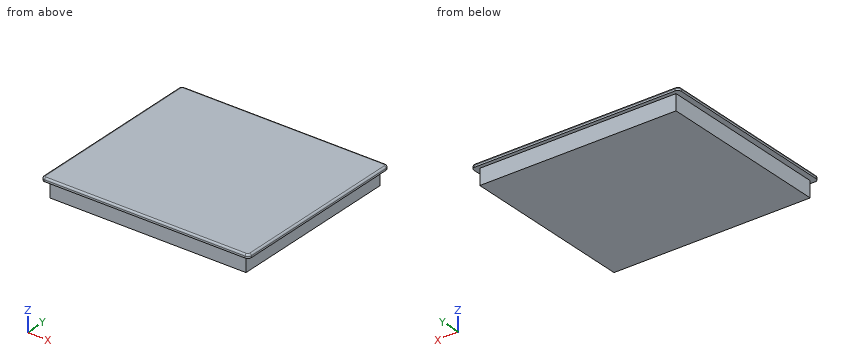
```python
from build123d import *

# Parameters (mm, degrees)
F0_W     = 560
F0_H     = 500
F1_DEPTH = 55
F2_DEPTH = 10
F3_R     = 5


with BuildPart() as f1:
    # F0 (on Top) → F1 (new body)
    with BuildSketch(Plane.XY):
        Rectangle(F0_W, F0_H)
    extrude(amount=-F1_DEPTH)

    # F0 (on Top) → F2 (join)
    with BuildSketch(Plane.XY):
        with BuildLine():
            Line((286, 261), (-286, 261))
            ThreePointArc((-286, 261), (-293.071068, 258.071068), (-296, 251))
            Line((-296, 251), (-296, -251))
            ThreePointArc((-296, -251), (-293.071068, -258.071068), (-286, -261))
            Line((-286, -261), (286, -261))
            ThreePointArc((286, -261), (293.071068, -258.071068), (296, -251))
            Line((296, -251), (296, 251))
            ThreePointArc((296, 251), (293.071068, 258.071068), (286, 261))
        make_face()
        Rectangle(F0_W, F0_H, mode=Mode.SUBTRACT)
        Rectangle(F0_W, F0_H)
    extrude(amount=-F2_DEPTH)

    # F3
    f3_edges = [f1.edges().sort_by_distance(p)[0] for p in [
        (0, 261, 0),
        (-293.071068, 258.071068, 0),
        (-296, 0, 0),
        (-293.071068, -258.071068, 0),
        (0, -261, 0),
        (293.071068, -258.071068, 0),
        (296, 0, 0),
        (293.071068, 258.071068, 0),
    ]]
    fillet(f3_edges, radius=F3_R)


solid = f1.part
```
For this review, take the finished solid that the model builds, in its own axes (mm). Round coordinates to 2 decimals unless told otherwise and drop trailing zeros. Write each loop counter-clockwise with the first axis right and the second up, starting at its lowest first coordinate (ties: lowest second). Pieces come first, ordered by that corner, then holes. Notation, with made-up numbers: (4, 23) -> (38, 23) arc R31 cw to (38, 58) -> close; hole circle Ø1 at (80.5, 4). An arc over 180 degrees is marked (long way). One line per question, with ' | ' between items. Start each with the question number.
1) Add section A-A (x = -79). Write out the cut boundary in (y, z).
2) For pin 1 Ø3 at (x, z) = (-74, -22.5) entering from +Y; pin 2 Ø10 at (y, z) = (-145.5, -35) entering from -X; pin 3 Ø1 at (x, z) = (105, -39.5) entering from -Y, all flat-tipped, find the tip position at first contact; note any pin that passes through.
3) Wall thickness on line 1 along Y through (x, z) = (-187, -38); line 2 along X through (y, z) = (201.5, -41); line 3 along Y through (x, z) = (184.5, -3): over which ranges is each line inside the solid? List them lowest first.
4) Add section C-C (z = -30.5). Write out the cut boundary in (x, y), and give its area (3 significant figures).
5) Add section B-B (y = -225). Write out the cut boundary in (x, z), and give its area (3 significant figures).
Reported:
1) outline: (-261, -10) -> (-250, -10) -> (-250, -55) -> (250, -55) -> (250, -10) -> (261, -10) -> (261, -5) arc R5 ccw to (256, 0) -> (-256, 0) arc R5 ccw to (-261, -5) -> close
2) pin 1: stops at y = 250 | pin 2: stops at x = -280 | pin 3: stops at y = -250
3) line 1: y = -250 to 250 | line 2: x = -280 to 280 | line 3: y = -260.58 to 260.58
4) outline: (-280, -250) -> (280, -250) -> (280, 250) -> (-280, 250) -> close | area: 280,000 mm²
5) outline: (-296, -10) -> (-280, -10) -> (-280, -55) -> (280, -55) -> (280, -10) -> (296, -10) -> (296, -5) arc R5 ccw to (291, 0) -> (-291, 0) arc R5 ccw to (-296, -5) -> close | area: 31,100 mm²
